from build123d import *

# Parameters (mm, degrees)
SKETCH1_W          = 464.185
SKETCH1_H          = 15.24
BASE_FLANGE1_DEPTH = 3.175
EDGE_FLANGE1_DEPTH = 464.185


# Sheet-metal steps are written as plain solids
with BuildPart() as part:
    # Sketch1 → Base-Flange1 (new body)
    with BuildSketch(Plane(origin=(0, 0, 0), x_dir=(1, 0, 0), z_dir=(0, 1, 0))):
        Rectangle(SKETCH1_W, SKETCH1_H)
    extrude(amount=-BASE_FLANGE1_DEPTH)

    # Edge-Flange1 section (across the edge) → Edge-Flange1 (add)
    with BuildSketch(Plane(origin=(-232.0925, 0, 8.89), x_dir=(0, 0, -1), z_dir=(1, 0, 0))):
        with BuildLine():
            Line((-3.175, 1), (-3.175, 15.24))
            Line((-3.175, 15.24), (0, 15.24))
            Line((0, 15.24), (0, 1))
            ThreePointArc((0, 1), (0.292893219, 0.292893219), (1, 0))
            Line((1, 0), (1.27, 0))
            Line((1.27, 0), (1.27, -3.175))
            Line((1.27, -3.175), (1, -3.175))
            ThreePointArc((1, -3.175), (-1.952170811, -1.952170811), (-3.175, 1))
        make_face()
    extrude(amount=EDGE_FLANGE1_DEPTH)


solid = part.part
The listing builds one solid part. Answer for the finished solid, in the listing's coordinates (mm). A direction names the side the tool comes from. Coordinates: 2 decimals unless noted, no trailing zeros. Loops run counter-clockwise (first coordinate to the right, second up) from the corner with the lowest first, then second, coordinate; pieces in that order, holes last.
1) Find section A-A on x = 62.5. Write down the section's boundary in (y, z) (3 decimals), then the cut area to 3 significant figures.
2) Find section C-C on z = -0.25. Write down the section's boundary in (x, y) (1 decimal), then the cut area to 3 significant figures.
3) Find section B-B on y = 4.25. Write down the section's boundary in (x, z) (1 decimal).
4) Flat-ended cylindrical pins translate along their axes: pin 1 Ø7 at (x, y) = (-26.5, 8) entering from -Z; pin 2 Ø4.5 at (x, z) = (104, 2.5) entering from +Y. Find the tip coordinate at first contact, or state that the pin passes through.
5) Find the intervals of material crossed by L1, parallel to Z at x = -197, y = 11.5 (3 decimals); L2, parallel to Y at x = 39.5, z = 6.75 (3 decimals); L3, parallel to Z at x = 41, y = -1.5, in increasing order.
6) A tool of negligible diameter and unlimited length cuts with its end or side. For faces 1 (the face through (-3, 8, 12.065)), 2 (the face through (-3, 8, 8.89)), from which of +Z, -Z, +X, -X, +Y, -Y can it reach the whole face along a straight path? Write none if from no direction.
Values:
1. outline: (-3.175, -7.62) - (0, -7.62) - (0, 7.89) arc R1 cw to (1, 8.89) - (15.24, 8.89) - (15.24, 12.065) - (1, 12.065) arc R4.175 ccw to (-3.175, 7.89) - close
1. area: 107 mm2
2. outline: (-232.1, -3.2) - (232.1, -3.2) - (232.1, 0) - (-232.1, 0) - close
2. area: 1,470 mm2
3. outline: (-232.1, 8.9) - (232.1, 8.9) - (232.1, 12.1) - (-232.1, 12.1) - close
4. pin 1: stops at z = 8.89
4. pin 2: stops at y = 0
5. L1: z = 8.89 to 12.065
5. L2: y = -3.175 to 0
5. L3: z = -7.62 to 11.23
6. face 1: +Z, +X, -X, +Y, -Y
6. face 2: -Z, +X, -X, +Y
